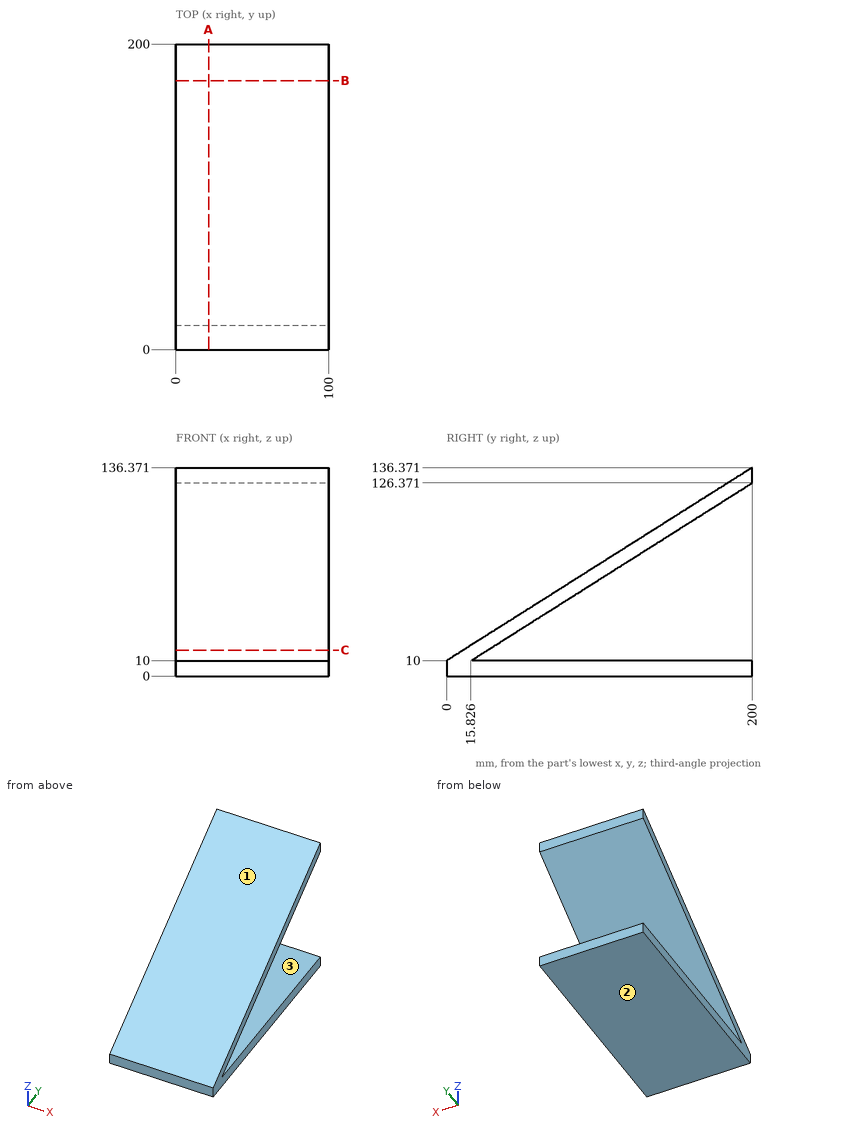
For this review, use the dimensioned drawing (mm, ordinates from the lowest corner) and the shaded views. Give positions to 0.01 mm unless a question says otherwise; leave off trailing zeros. Loops run counter-clockwise (first coordinate to the right, second up) from the corner with the lowest first, then second, coordinate; pieces in that order, holes last. Notation, with made-up numbers: (12.5, 58.25) -> (46.5, 58.25) arc R25 ccw to (46.5, 97.25) -> close; hole circle Ø8 at (26, 87.5). An arc over 180 degrees is marked (long way). Use CSV: the item, a comma, the result in double quotes.
1. Consider section C-C, the plane z = 17. Write out the cut boundary in (x, y) (1 decimal).
Result:
outline,"(0, 11.1) -> (100, 11.1) -> (100, 26.9) -> (0, 26.9) -> close"
2. For P1, Ø1.5, axis at x = 60.5, z = 100, coming from the -Y side; P2, Ø1.5, axis at x = 14, y = 176, coming from the +Z side, all flat-tipped, find the tip position at first contact; note any pin that passes through.
Result:
P1,"stops at y = 141.25"
P2,"stops at z = 121.68"
3. To check wall thickness, follow probe 1 along Z at (x, y) = (71, 175) (1 decimal); probe 2 along Z at (x, y) = (71, 156.5) (1 decimal); probe 3 along Y at (x, z) = (34, 35.5) (1 decimal). State the ranges of each line that lie inside material, in increasing order. Write a range as from..to.
Result:
probe 1,"z = 0..10, 110.6..120.6"
probe 2,"z = 0..10, 98.9..108.9"
probe 3,"y = 40.4..56.2"
4. Consider section B-B, the plane y = 176. Write out the cut boundary in (x, z).
Result:
outline,"(0, 0) -> (100, 0) -> (100, 10) -> (0, 10) -> close; (0, 111.21) -> (100, 111.21) -> (100, 121.21) -> (0, 121.21) -> close"
5. The part is to be moulded in two halves that separate along Z. For the marked faces 1, 2 and 3, say which applies: +Z half, -Z half, draft (parallel to the pull), parting line (faces both ways), or undercut.
Result:
face 1,"+Z half"
face 2,"-Z half"
face 3,"undercut"
6. Consider section A-A, the plane x = 21.5. Write out the cut boundary in (y, z).
Result:
outline,"(0, 0) -> (200, 0) -> (200, 10) -> (15.83, 10) -> (200, 126.37) -> (200, 136.37) -> (0, 10) -> close"
